Source: CAD feature listing. Evaluate the final solid. Frame: model axes, mm. Coordinates: 2 decimals unless noted, no trailing zeros. Order: outer loops, then holes, each group sorted by start corner. A loop starts at its lowest first (then second) coordinate and runs counter-clockwise, first axis right, second up.
```python
from build123d import *

# Parameters (mm, degrees)
SKETCH6_R           = 1.5
BOSS_EXTRUDE4_DEPTH = 6
CIRPATTERN1_COUNT   = 3
SKETCH8_W           = 3
SKETCH8_H           = 50
CUT_EXTRUDE3_DEPTH  = 7
CUT_EXTRUDE4_DEPTH  = 7
FILLET1_R           = 10
FILLET2_R           = 5
SKETCH9_W           = 25
SKETCH9_H           = 3
CUT_EXTRUDE5_DEPTH  = 7


with BuildPart() as part:
    # Sketch6 → Boss-Extrude4 (new body)
    with BuildSketch(Plane(origin=(0, 0, 0), x_dir=(1, 0, 0), z_dir=(0, 1, 0))):
        Polygon((0, 0), (55.980762114, 96.961524227), (120, 60), (120, -60), (55.980762114, -96.961524227), align=None)
        with Locations((95, 55)):
            Circle(SKETCH6_R, mode=Mode.SUBTRACT)
        with Locations((110, 55)):
            Circle(SKETCH6_R, mode=Mode.SUBTRACT)
        with Locations((95, -55)):
            Circle(SKETCH6_R, mode=Mode.SUBTRACT)
        with Locations((110, -55)):
            Circle(SKETCH6_R, mode=Mode.SUBTRACT)
    boss_extrude4 = extrude(amount=BOSS_EXTRUDE4_DEPTH)

    # CirPattern1: Boss-Extrude4 ×3 about axis
    cirpattern1_axis = Axis((0, 0, 0), (0, 1, 0))
    for i in range(1, CIRPATTERN1_COUNT):
        add(boss_extrude4.rotate(cirpattern1_axis, i * 360 / CIRPATTERN1_COUNT))

    # Sketch8 → Cut-Extrude3 (cut, through all)
    with BuildSketch(Plane(origin=(0, 6, 0), x_dir=(1, 0, 0), z_dir=(0, 1, 0))):
        Polygon((73.612159322, -77.5), (30.310889132, -102.5), (28.810889132, -99.901923789), (72.112159322, -74.901923789), align=None)
        with Locations((102.423048454, 0)):
            Rectangle(SKETCH8_W, SKETCH8_H)
        Polygon((-30.310889132, -102.5), (-73.612159322, -77.5), (-72.112159322, -74.901923789), (-28.810889132, -99.901923789), align=None)
        with Locations((-102.423048454, 0)):
            Rectangle(SKETCH8_W, SKETCH8_H)
        Polygon((-73.612159322, 77.5), (-30.310889132, 102.5), (-28.810889132, 99.901923789), (-72.112159322, 74.901923789), align=None)
        Polygon((30.310889132, 102.5), (73.612159322, 77.5), (72.112159322, 74.901923789), (28.810889132, 99.901923789), align=None)
    extrude(amount=-CUT_EXTRUDE3_DEPTH, mode=Mode.SUBTRACT)

    # Sketch7 → Cut-Extrude4 (cut, through all)
    with BuildSketch(Plane(origin=(0, 6, 0), x_dir=(1, 0, 0), z_dir=(0, 1, 0))):
        Polygon((-61.961524227, 45.055534995), (-61.961524227, -45.055534995), (-8.038475773, -76.188021535), (70, -31.132486541), (70, 31.132486541), (-8.038475773, 76.188021535), align=None)
    extrude(amount=-CUT_EXTRUDE4_DEPTH, mode=Mode.SUBTRACT)

    # Fillet1
    fillet1_edges = [part.edges().sort_by_distance(p)[0] for p in [
        (-61.961524227, 3, -45.055534995),
        (-8.038475773, 3, -76.188021535),
        (70, 3, -31.132486541),
        (70, 3, 31.132486541),
        (-8.038475773, 3, 76.188021535),
        (-61.961524227, 3, 45.055534995),
    ]]
    fillet(fillet1_edges, radius=FILLET1_R)

    # Fillet2
    fillet2_edges = [part.edges().sort_by_distance(p)[0] for p in [
        (-8.038475773, 3, -133.923048454),
        (-111.961524227, 3, -73.923048454),
        (-111.961524227, 3, 73.923048454),
        (-8.038475773, 3, 133.923048454),
        (120, 3, -60),
        (120, 3, 60),
    ]]
    fillet(fillet2_edges, radius=FILLET2_R)

    # Sketch9 → Cut-Extrude5 (cut, through all)
    with BuildSketch(Plane(origin=(0, 6, 0), x_dir=(1, 0, 0), z_dir=(0, 1, 0))):
        with Locations((102.423048454, -25)):
            Rectangle(SKETCH9_W, SKETCH9_H)
        with Locations((102.423048454, 25)):
            Rectangle(SKETCH9_W, SKETCH9_H)
        Polygon((-67.911197427, -64.625644347), (-65.313121216, -66.125644347), (-77.813121216, -87.776279442), (-80.411197427, -86.276279442), align=None)
        Polygon((-24.609927238, -89.625644347), (-22.011851027, -91.125644347), (-34.511851027, -112.776279442), (-37.109927238, -111.276279442), align=None)
        Polygon((-22.011851027, 91.125644347), (-24.609927238, 89.625644347), (-37.109927238, 111.276279442), (-34.511851027, 112.776279442), align=None)
        Polygon((-65.313121216, 66.125644347), (-67.911197427, 64.625644347), (-80.411197427, 86.276279442), (-77.813121216, 87.776279442), align=None)
    extrude(amount=-CUT_EXTRUDE5_DEPTH, mode=Mode.SUBTRACT)


solid = part.part
```
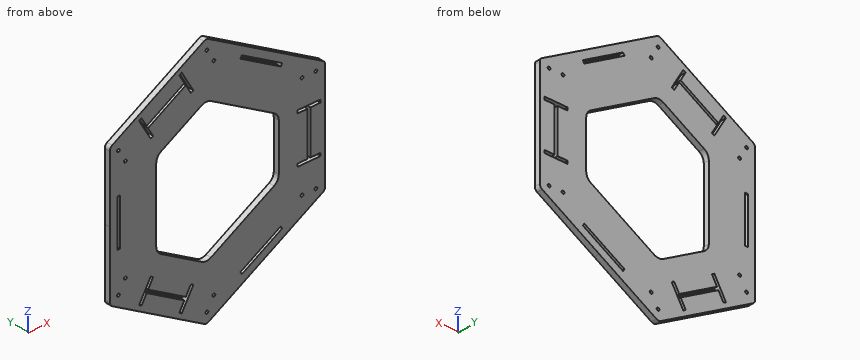
1. Contact query for flat-ended pins moving along their axis: P1, Ø1.5, axis at x = -102, y = 2.5, coming from the +Z side; P2, Ø1.5, axis at x = 46.5, y = 5, coming from the -Z side; P3, Ø1.5, axis at x = -102, y = 2.5, coming from the -Z side. Output: stop coordinate, or through.
2. Section query C-C, the plane x = 7. Output: boundary loops of the cut face in (y, z), plus the area to 3 significant figures.
3. Section query B-B, the plane z = 6. Output: boundary loops of the cut face in (x, y).
4. Section query D-D, the plane y = 4. Count the separate pieces of the cut face and the enclosed holes in it, plus the area to 3 significant figures.
5. Section query A-A, the plane z = -29.5. Output: boundary loops of the cut face in (x, y).
6. Material intervals for line 1 along X through (y, z) = (1.25, 21); line 2 along Z through (x, y) = (90, 2.5); line 3 along X through (y, z) = (3.5, 65.5), sorted ascending.
Answer key:
1. P1: stops at z = 80.11
1. P2: stops at z = -102.87
1. P3: stops at z = -80.11
2. outline: (0, -125.24) - (6, -125.24) - (6, -67.51) - (0, -67.51) - close; (0, 67.51) - (6, 67.51) - (6, 125.24) - (0, 125.24) - close
2. area: 693 mm2
3. outline: (-111.96, 0) - (-103.92, 0) - (-103.92, 6) - (-111.96, 6) - close; (-100.92, 0) - (-61.96, 0) - (-61.96, 6) - (-100.92, 6) - close; (70, 0) - (100.92, 0) - (100.92, 6) - (70, 6) - close; (103.92, 0) - (120, 0) - (120, 6) - (103.92, 6) - close
4. separate pieces: 1
4. enclosed holes: 19
4. area: 30,100 mm2
5. outline: (-111.96, 0) - (-61.96, 0) - (-61.96, 6) - (-111.96, 6) - close; (69.1, 0) - (120, 0) - (120, 6) - (69.1, 6) - close
6. line 1: x = -111.96 to -103.92, -100.92 to -61.96, 70 to 100.92, 103.92 to 120
6. line 2: z = -77.32 to -26.5, -23.5 to 23.5, 26.5 to 77.32
6. line 3: x = -111.96 to -68.42, -66.4 to -26.55, 10.47 to 110.47
